Autodesk Inventor part; units mm, degrees
ref_plane "YZ Plane" through (0, 0, 0) normal (1, 0, 0) x (0, 1, 0)
ref_plane "XZ Plane" through (0, 0, 0) normal (0, 1, 0) x (-1, 0, 0)
ref_plane "XY Plane" through (0, 0, 0) normal (0, 0, 1) x (1, 0, 0)
sketch "草圖1" plane through (0, 0, 0) normal (1, 0, 0) x (0, 1, 0)
  line L0 (-8.5, 0) -> (-8.5, -8)
  line L1 (-8.5, -8) -> (-6.5, -8)
  line L2 (-6.5, -8) -> (-6.5, -4)
  line L3 (-6.5, -4) -> (-3.5, -4)
  line L4 (3.5, -4) -> (3.5, -8)
  line L5 (3.5, -8) -> (-3.5, -8)
  line L6 (8.5, 0) -> (8.5, -8)
  line L7 (8.5, -8) -> (6.5, -8)
  line L8 (6.5, -8) -> (6.5, -4)
  line L9 (6.5, -4) -> (3.5, -4)
  line L10 (8.5, 0) -> (-8.5, 0)
  line L11 (-3.5, -8) -> (-3.5, -4)
  point P0 (0, 0)
  point P1 (0, 0)
  point P2 (0, 0)
  dimension "d2" = 3
  dimension "d3" = 7
  dimension "d4" = 8
  dimension "d5" = 4
  dimension "d6" = 2
  dimension "d12" = 17
extrude "擠出1" add sketch "草圖1" along normal blind 3
fillet "圓角1" radius 2 2 edges at (1.5, 8.5, 0) (1.5, -8.5, 0)
fillet "圓角2" radius 1 4 edges at (1.5, 6.5, -8) (1.5, 3.5, -8) (1.5, -3.5, -8) (1.5, -6.5, -8)
fillet "圓角3" radius 1 2 edges at (1.5, 8.5, -8) (1.5, -8.5, -8)
properties part number "support" material "木材 (楓木)"
Model file for the job. Use its own axes, mm. A direction names the side the tool comes from. Round coordinates to 2 decimals unless told otherwise and drop trailing zeros. Order: outer loops, then holes, each group sorted by start corner. A loop starts at its lowest first (then second) coordinate and runs counter-clockwise, first axis right, second up.
(1) Pull direction Y, two halves, no side cores. Call faces 3 (the face through (1, -5, -4)), 4 (the face through (1.521, -8.215, -7.699)), 5 (the face through (1, 0, 0)), 6 (the face through (1.52, 7.93, -0.6)): released by +Y, released by -Y, zero draft, split by the parting line, or undercut.
(2) Band-saw the part on C-C (y = 4.75). List the corners of the cut face in (x, z).
(3) Band-saw the part on A-A (z = -4.75). List the corners of the cut face in (x, y), then the cut area to 3 significant figures.
(4) 3-axis set-ups, long thin cutter, end or side, ignore diameter. For faces 1 (the face through (0, 0, -3)), 2 (the face through (1.521, -6.801, -7.715)): which of +Z, -Z, +X, -X, +Y, -Y reach the whole face in a straight line?
(5) Drill centre lines: line 1 (Y direction, x = 1.45, z = -4.5); line 2 (Z direction, x = 1.7, y = 3.75); line 3 (Y direction, x = 1.3, z = -1.75). Where is each one in solid material? Low to high.
(6) Pin check, flat tip, straight feed: pin 1 (0.9 mm diameter, centred on x = 2, y = -4.5, fed in from -Z). Stop position of the tip, or through.
Verdict:
1. face 3: undercut
1. face 4: released by -Y
1. face 5: zero draft
1. face 6: released by +Y
2. outline: (0, -4) - (3, -4) - (3, 0) - (0, 0) - close
3. outline: (0, -8.5) - (3, -8.5) - (3, -6.5) - (0, -6.5) - close; (0, -3.5) - (3, -3.5) - (3, 3.5) - (0, 3.5) - close; (0, 6.5) - (3, 6.5) - (3, 8.5) - (0, 8.5) - close
3. area: 33.0 mm2
4. face 1: +Z, -Z, -X, +Y, -Y
4. face 2: -Z, +X, -X
5. line 1: y = -8.5 to -6.5, -3.5 to 3.5, 6.5 to 8.5
5. line 2: z = -4 to 0
5. line 3: y = -8.48 to 8.48
6. pin 1: stops at z = -4
